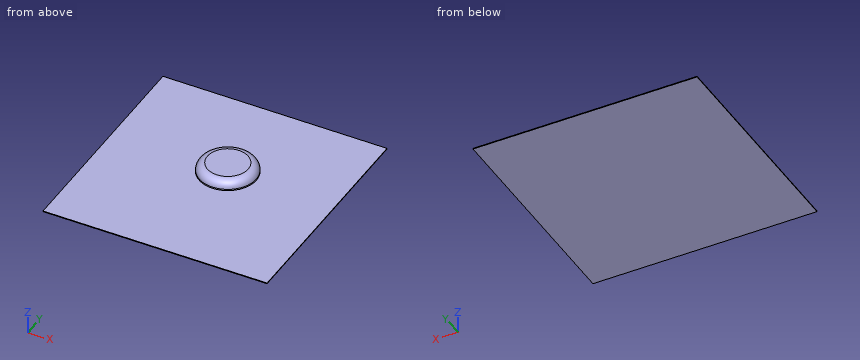
from build123d import *

# Parameters (mm, degrees)
SKETCH006_W  = 11
SKETCH006_H  = 11
PAD003_DEPTH = 0.0348
SKETCH007_R  = 1.4
PAD004_DEPTH = 0.5
FILLET_R     = 0.4


with BuildPart() as part:
    # Sketch006 → Pad003 (new body)
    with BuildSketch(Plane.XY):
        Rectangle(SKETCH006_W, SKETCH006_H)
    extrude(amount=PAD003_DEPTH)

    # Sketch007 → Pad004 (join)
    with BuildSketch(Plane.XY):
        with Locations((0.2, 0.8)):
            Circle(SKETCH007_R)
    extrude(amount=PAD004_DEPTH)

    # Fillet
    fillet_edges = [part.edges().sort_by_distance(p)[0] for p in [
        (-1.2, 0.8, 0.5),
    ]]
    fillet(fillet_edges, radius=FILLET_R)


with BuildPart() as part_1:
    # Body003 placement: moved
    add(part.part.moved(Location((0, 0, 4.7))))


solid = part_1.part
Input: part model. Units: mm. Frame: model coordinates. Coordinates: 2 decimals unless noted, no trailing zeros. Order: outer loops, then holes, each group sorted by start corner. A loop starts at its lowest first (then second) coordinate and runs counter-clockwise, first axis right, second up. Notation, with made-up numbers: M -5.75,25 L 29.25,25 A16 ccw 29.25,50 Z; hole C -2.5,-10 d2. An arc over 180 degrees is marked long. Answer in a Markdown table with one row per item.
(1) Material intervals for line 1 (X direction, y = 0.25, z = 4.95); line 2 (Y direction, x = 0, z = 5.1); line 3 (Y direction, x = 0.5, z = 4.9), sorted ascending. Write a range as [from, to].
Numbers:
| item | result |
|---|---|
| line 1 | x = [-1.06, 1.46] |
| line 2 | y = [-0.45, 2.05] |
| line 3 | y = [-0.55, 2.15] |
(2) Contact query for flat-ended pins moving along their axis: pin 1 Ø1 at (x, y) = (0.5, 3) entering from +Z; pin 2 Ø6 at (x, y) = (-1, 1) entering from +Z. Output: stop coordinate, or through.
Numbers:
| item | result |
|---|---|
| pin 1 | stops at z = 4.73 |
| pin 2 | stops at z = 5.2 |
(3) Section query D-D, the plane z = 4.9. Output: boundary loops of the cut face in (x, y).
Numbers:
| item | result |
|---|---|
| outline | C 0.2,0.8 d2.77 |
